```python
from build123d import *

# Parameters (mm, degrees)
SKETCH1_W           = 48.49
SKETCH1_H           = 38.3
BOSS_EXTRUDE1_DEPTH = 8.705
FILLET1_R           = 7
FILLET2_R           = 3
FILLET3_R           = 1


with BuildPart() as part:
    # Sketch1 → Boss-Extrude1 (new, symmetric)
    with BuildSketch(Plane(origin=(0, 0, 0), x_dir=(1, 0, 0), z_dir=(0, 1, 0))):
        Rectangle(SKETCH1_W, SKETCH1_H)
    extrude(amount=BOSS_EXTRUDE1_DEPTH, both=True)

    # Fillet1
    fillet1_edges = [part.edges().sort_by_distance(p)[0] for p in [
        (24.245, 0, 19.15),
        (-24.245, 0, 19.15),
        (-24.245, 0, -19.15),
        (24.245, 0, -19.15),
    ]]
    fillet(fillet1_edges, radius=FILLET1_R)

    # Fillet2
    fillet2_edges = [part.edges().sort_by_distance(p)[0] for p in [
        (-24.245, 8.705, 0),
        (0, 8.705, -19.15),
        (24.245, 8.705, 0),
        (0, 8.705, 19.15),
        (-22.194747468, 8.705, 17.099747468),
        (22.194747468, 8.705, 17.099747468),
        (22.194747468, 8.705, -17.099747468),
        (-22.194747468, 8.705, -17.099747468),
    ]]
    fillet(fillet2_edges, radius=FILLET2_R)

    # Fillet3
    fillet3_edges = [part.edges().sort_by_distance(p)[0] for p in [
        (-24.245, -8.705, 0),
        (24.245, -8.705, 0),
        (0, -8.705, 19.15),
        (0, -8.705, -19.15),
        (-22.194747468, -8.705, 17.099747468),
        (22.194747468, -8.705, 17.099747468),
        (22.194747468, -8.705, -17.099747468),
        (-22.194747468, -8.705, -17.099747468),
    ]]
    fillet(fillet3_edges, radius=FILLET3_R)


solid = part.part
```
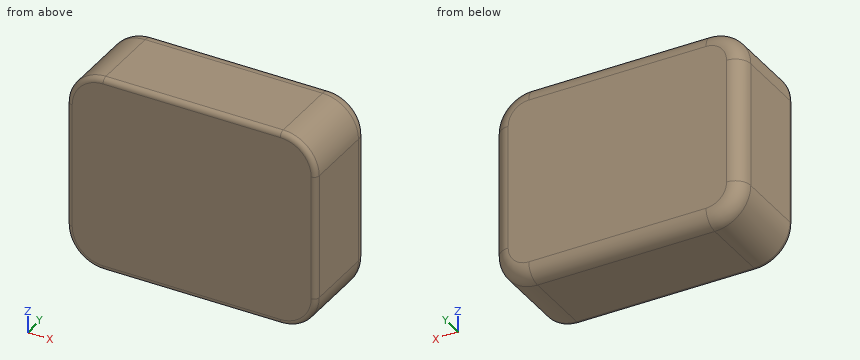
Verification items for the finished model (mm, model axes). Round coordinates to 2 decimals unless told otherwise and drop trailing zeros. Order: outer loops, then holes, each group sorted by start corner. A loop starts at its lowest first (then second) coordinate and runs counter-clockwise, first axis right, second up. Notation, with made-up numbers: (-35.5, 17.5) -> (-15.5, 17.5) arc R15 ccw to (-15.5, 21.5) -> close; hole circle Ø6 at (89.25, -31.5). An arc over 180 degrees is marked (long way). Put each result on its own line as item: value. Start each with the question number.
(1) Depth check by flat-ended pin: pin 1 Ø6 at (y, z) = (6.5, 6.5) entering from +X (3 decimals). Enter the tip coordinate at first touch or a pass-through.
(2) Material ranges on line 1 along X through (y, z) = (1, -14.5); line 2 along X through (y, z) = (-1.5, -15); line 3 along Y through (x, z) = (-18, -17) (3 decimals), recorded low to high.
(3) Section check A-A (y = -4). Enter the section's corners in (x, z) (3 decimals).
Completed:
1. pin 1: stops at x = 24.245
2. line 1: x = -23.84 to 23.84
2. line 2: x = -23.64 to 23.64
2. line 3: y = -8.705 to 8.564
3. outline: (-24.245, -12.15) arc R7 ccw to (-17.245, -19.15) -> (17.245, -19.15) arc R7 ccw to (24.245, -12.15) -> (24.245, 12.15) arc R7 ccw to (17.245, 19.15) -> (-17.245, 19.15) arc R7 ccw to (-24.245, 12.15) -> close
